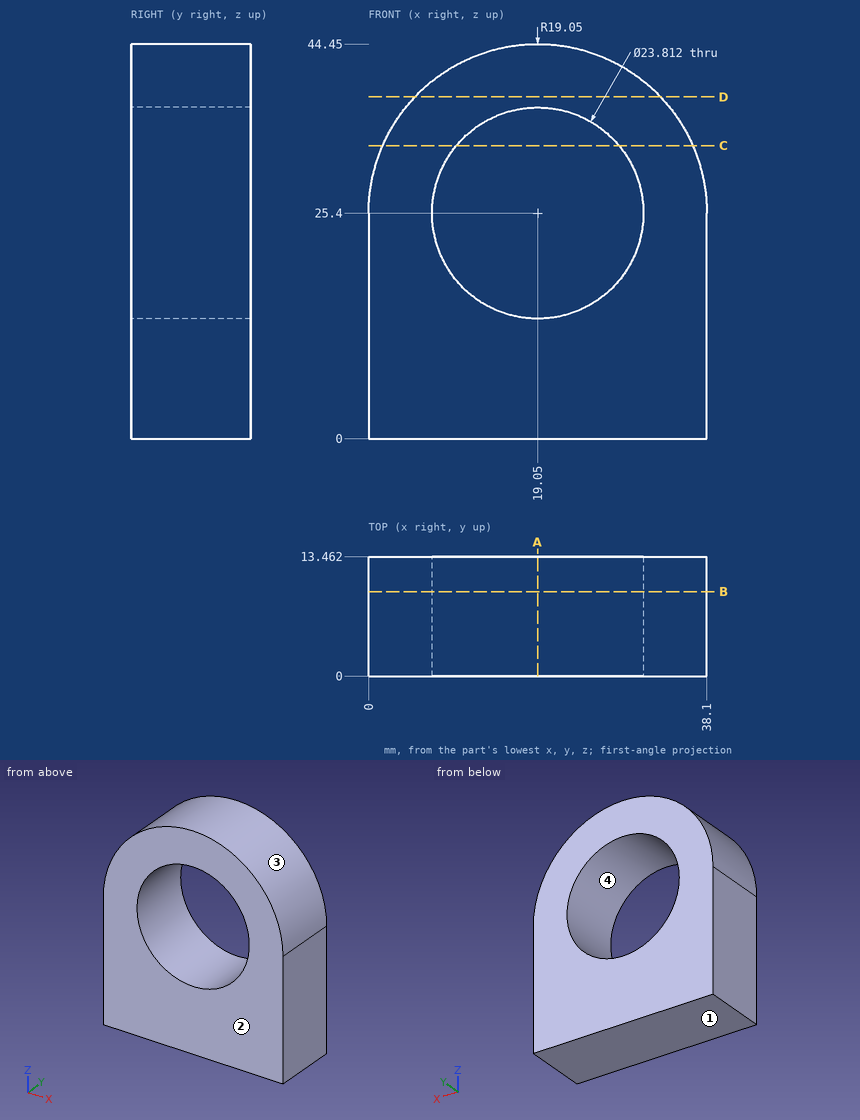
Print and shaded views of the part. All mm, measured from the part's lowest x, y and z. Round coordinates to 2 decimals unless told otherwise and drop trailing zeros. Write each loop counter-clockwise with the first axis right and the second up, starting at its lowest first coordinate (ties: lowest second). Pieces come first, ordered by that corner, then holes. Notation, with made-up numbers: (39, 36.5) - (43, 36.5) arc R30 cw to (43, 60.5) - close; hole circle Ø4 at (-4.75, 45). An arc over 180 degrees is marked (long way). Write each question's results on one line, items separated by ' | '. Start each with the question number.
Item 1: Mould opens along Z. For the marked faces 1, 2, 3 and 4 say: pulls with the +Z half, pulls with the -Z half, needs draft (parallel to the pull), parting line crosses it, or undercut.
Item 2: Wall check: L1, parallel to Z at x = 19.05, y = 3.25; L2, parallel to Z at x = 27, y = 12.25 (1 decimal); L3, parallel to X at y = 10.75, z = 29. Give the ranges that are in metal, low to high. Write a range as [from, to].
Item 3: Saw through at A-A (x = 19.05). Write the cut outline in (y, z).
Item 4: Saw through at C-C (z = 33). Write the cut outline in (x, y) (1 decimal).
Item 5: Saw through at D-D (z = 38.5). Write the cut outline in (x, y), and give its area (3 significant figures).
Item 6: Drop flat-ended pins along their axis: P1, Ø4, axis at y = 1.5, z = 35.5, coming from the -X side; P2, Ø4, axis at x = 12, z = 19.5, coming from the +Y side. Give the stop position or say it passes through.
Item 7: Saw through at B-B (y = 9.5). Write the cut outline in (x, z), and give its area (3 significant figures).
Results are:
1) face 1: pulls with the -Z half | face 2: needs draft | face 3: pulls with the +Z half | face 4: undercut
2) L1: z = [0, 13.49], [37.31, 44.45] | L2: z = [0, 16.5], [34.3, 42.7] | L3: x = [0.34, 7.7], [30.4, 37.76]
3) outline: (0, 0) - (13.46, 0) - (13.46, 13.49) - (0, 13.49) - close; (0, 37.31) - (13.46, 37.31) - (13.46, 44.45) - (0, 44.45) - close
4) outline: (1.6, 0) - (9.9, 0) - (9.9, 13.5) - (1.6, 13.5) - close; (28.2, 0) - (36.5, 0) - (36.5, 13.5) - (28.2, 13.5) - close
5) outline: (5.22, 0) - (32.88, 0) - (32.88, 13.46) - (5.22, 13.46) - close | area: 372 mm²
6) P1: stops at x = 1.81 | P2: passes through
7) outline: (0, 0) - (38.1, 0) - (38.1, 25.4) arc R19.05 ccw to (0, 25.4) - close; hole circle Ø23.81 at (19.05, 25.4) | area: 1,090 mm²
